Check sheet for the modelled part. Datum: model origin and axes. Units: mm. A direction names the side the tool comes from. Give positions to 0.01 mm unless a question says otherwise; leave off trailing zeros. Order: outer loops, then holes, each group sorted by start corner. A loop starts at its lowest first (then second) coordinate and runs counter-clockwise, first axis right, second up. Notation, with made-up numbers: M 12,-11.75 L 35,-11.75 A20 cw 35,21.25 Z; hole C -2,33.25 d11. An arc over 180 degrees is marked long. Return JSON: item names as keys, results as strings. Group by question number.
from build123d import *

# Parameters (mm, degrees)
BOX301_W        = 7
BOX301_H        = 2.3
BOX301_DEPTH    = 5
FILLET223_R     = 0.3
CHAMFER043_SIZE = 1.3
CHAMFER044_SIZE = 1.3
BOX300_W        = 7.3
BOX300_H        = 2.6
BOX300_DEPTH    = 5.5
FILLET222_R     = 0.3
CHAMFER041_SIZE = 1.3
CHAMFER042_SIZE = 1.3
BOX302_W        = 5
BOX302_H        = 0.5
BOX302_DEPTH    = 4


with BuildPart() as chamfer044:
    # Box301 → Box301 (new body)
    with BuildSketch(Plane.XY):
        with Locations((3.5, 1.15)):
            Rectangle(BOX301_W, BOX301_H)
    extrude(amount=BOX301_DEPTH)

    # Fillet223
    fillet223_edges = [chamfer044.edges().sort_by_distance(p)[0] for p in [
        (0, 0, 2.5),
        (7, 0, 2.5),
    ]]
    fillet(fillet223_edges, radius=FILLET223_R)

    # Chamfer043
    chamfer043_edges = [chamfer044.edges().sort_by_distance(p)[0] for p in [
        (7, 2.3, 2.5),
    ]]
    chamfer(chamfer043_edges, length=CHAMFER043_SIZE)

    # Chamfer044
    chamfer044_edges = [chamfer044.edges().sort_by_distance(p)[0] for p in [
        (0, 2.3, 2.5),
    ]]
    chamfer(chamfer044_edges, length=CHAMFER044_SIZE)


with BuildPart() as chamfer044_1:
    # Chamfer044 placement: moved
    add(chamfer044.part.moved(Location((0.15, 0.15, 0))))


with BuildPart() as cut347:
    # Box300 → Box300 (new body)
    with BuildSketch(Plane.XY):
        with Locations((3.65, 1.3)):
            Rectangle(BOX300_W, BOX300_H)
    extrude(amount=BOX300_DEPTH)

    # Fillet222
    fillet222_edges = [cut347.edges().sort_by_distance(p)[0] for p in [
        (0, 0, 2.75),
        (7.3, 0, 2.75),
    ]]
    fillet(fillet222_edges, radius=FILLET222_R)

    # Chamfer041
    chamfer041_edges = [cut347.edges().sort_by_distance(p)[0] for p in [
        (7.3, 2.6, 2.75),
    ]]
    chamfer(chamfer041_edges, length=CHAMFER041_SIZE)

    # Chamfer042
    chamfer042_edges = [cut347.edges().sort_by_distance(p)[0] for p in [
        (0, 2.6, 2.75),
    ]]
    chamfer(chamfer042_edges, length=CHAMFER042_SIZE)

    # Cut347: cut Chamfer044
    add(chamfer044_1.part, mode=Mode.SUBTRACT)


with BuildPart() as obj1:
    # Box302 → Box302 (new body)
    with BuildSketch(Plane(origin=(1, 1, 1.5), x_dir=(1, 0, 0), z_dir=(0, 0, 1))):
        with Locations((2.5, 0.25)):
            Rectangle(BOX302_W, BOX302_H)
    extrude(amount=BOX302_DEPTH)

    # Fusion204: union Cut347
    add(cut347.part)


with BuildPart() as obj1_1:
    # Fusion204 placement: moved
    add(obj1.part.moved(Location((-14, -20.6, 2.5))))


solid = obj1_1.part
1) Sectioned sample at A-A on z = 6.85. Record the boundary of the cut face in (x, y), then the cut area to 3 significant figures.
2) Sectioned sample at C-C on y = -18.75. Record the boundary of the cut face in (x, z).
3) Release check for a two-part mould opening along Y. For faces 1 (the face through (-14, -20, 5)), 2 (the face through (-7, -19, 5)), 3 (the face through (-10, -20, 7.5)) record: released by +Y, released by -Y, zero draft, split by the parting line, or undercut.
4) Depth check by flat-ended pin: P1, Ø1.2, axis at x = -11, y = -19.5, coming from the -Z side; P2, Ø1, axis at y = -18.5, z = 3.5, coming from the +X side. Enter the tip coordinate at first touch or a pass-through.
5) Sectioned sample at D-D on x = -9. Record the boundary of the cut face in (y, z), then the cut area to 3 significant figures.
6) Sectioned sample at B-B on z = 3.7. Record the boundary of the cut face in (x, y).
7) Material ranges on line 1 along X through (y, z) = (-20.1, 4.65); line 2 along Z through (x, y) = (-7.75, -20.05); line 3 along X through (y, z) = (-18.6, 7.25), recorded low to high.
8) Tool access check on faces 4 (the face through (-13.2, -18.8, 5)), 5 (the face through (-10, -18, 5)). Record the directions out of +Z, -Z, +X, -X, +Y, -Y that give a thin tool (end or side, any length) a straight path to the whole face; none if there is none.
Reply:
{
 "1": {"outline": "M -14,-20.3 A0.3 ccw -13.7,-20.6 L -7,-20.6 A0.3 ccw -6.7,-20.3 L -6.7,-19.3 L -8,-18 L -12.7,-18 L -14,-19.3 Z; M -13,-19.6 L -8,-19.6 L -8,-19.1 L -13,-19.1 Z; hole M -13.85,-20.15 A0.3 ccw -13.55,-20.45 L -7.15,-20.45 A0.3 ccw -6.85,-20.15 L -6.85,-19.45 L -8.15,-18.15 L -12.55,-18.15 L -13.85,-19.45 Z", "area": "5.38 mm^2"},
 "2": {"outline": "M -13.45,2.5 L -13.15,2.5 L -13.15,7.5 L -7.55,7.5 L -7.55,2.5 L -7.25,2.5 L -7.25,8 L -13.45,8 Z"},
 "3": {"face 1": "zero draft", "face 2": "released by +Y", "face 3": "undercut"},
 "4": {"P1": "z = 4", "P2": "x = -7"},
 "5": {"outline": "M -20.6,2.5 L -20.45,2.5 L -20.45,7.5 L -19.6,7.5 L -19.6,4 L -19.1,4 L -19.1,7.5 L -18.15,7.5 L -18.15,2.5 L -18,2.5 L -18,8 L -20.6,8 Z", "area": "4.55 mm^2"},
 "6": {"outline": "M -14,-20.3 A0.3 ccw -13.7,-20.6 L -7,-20.6 A0.3 ccw -6.7,-20.3 L -6.7,-19.3 L -8,-18 L -12.7,-18 L -14,-19.3 Z; hole M -13.85,-20.15 A0.3 ccw -13.55,-20.45 L -7.15,-20.45 A0.3 ccw -6.85,-20.15 L -6.85,-19.45 L -8.15,-18.15 L -12.55,-18.15 L -13.85,-19.45 Z"},
 "7": {"line 1": "-14 to -13.85, -6.85 to -6.7", "line 2": "7.5 to 8", "line 3": "-13.3 to -13, -7.7 to -7.4"},
 "8": {"face 4": "-Z", "face 5": "+Z, -Z, +X, -X, +Y"}
}
